Geometry: see drawing. Coordinates: mm, zero at the bounding-box minimum. A direction names the side the tool comes from. Round coordinates to 2 decimals unless told otherwise and drop trailing zeros. Loops run counter-clockwise (first coordinate to the right, second up) from the corner with the lowest first, then second, coordinate; pieces in that order, holes last.
(1) Cut plane B-B, the plane y = 93.5. Output: boundary loops of the cut face in (x, z), and give its area (3 significant figures).
(2) Line query: line 1 (X direction, y = 96.5, z = 148); line 2 (X direction, y = 173, z = 15); line 3 (Y direction, x = 136, z = 57.5). Output: solid intervals per line, ascending.
(3) Access query for the marked faces 1, 2, 3 and 4. Directions: +Z, -Z, +X, -X, +Y, -Y. A direction counts if a zero-diameter tool reaches every point of the face in a straight line with its end or side. Return the directions, or none.
(4) Cut plane C-C, the plane x = 85. Output: boundary loops of the cut face in (y, z), and give its area (3 significant figures).
(5) First-contact query: pin 1 Ø10 at (y, z) = (62.5, 78) entering from +X; pin 2 Ø6 at (x, z) = (204.5, 25) entering from -Y; pin 3 Ø4 at (x, z) = (191.5, 154) entering from -Y. Flat tips, straight axial feed; report the tip coordinate or a pass-through.
(6) Cut plane A-A, the plane z = 51. Output: boundary loops of the cut face in (x, y), and give its area (3 significant figures).
(7) Cut plane D-D, the plane z = 92.5. Output: boundary loops of the cut face in (x, y), and give its area (3 significant figures).
(8) Draft query along X for the marked faces 5, 6, 7 and 8. Return one class per face: released by +X, released by -X, zero draft, split by the parting line, or undercut.
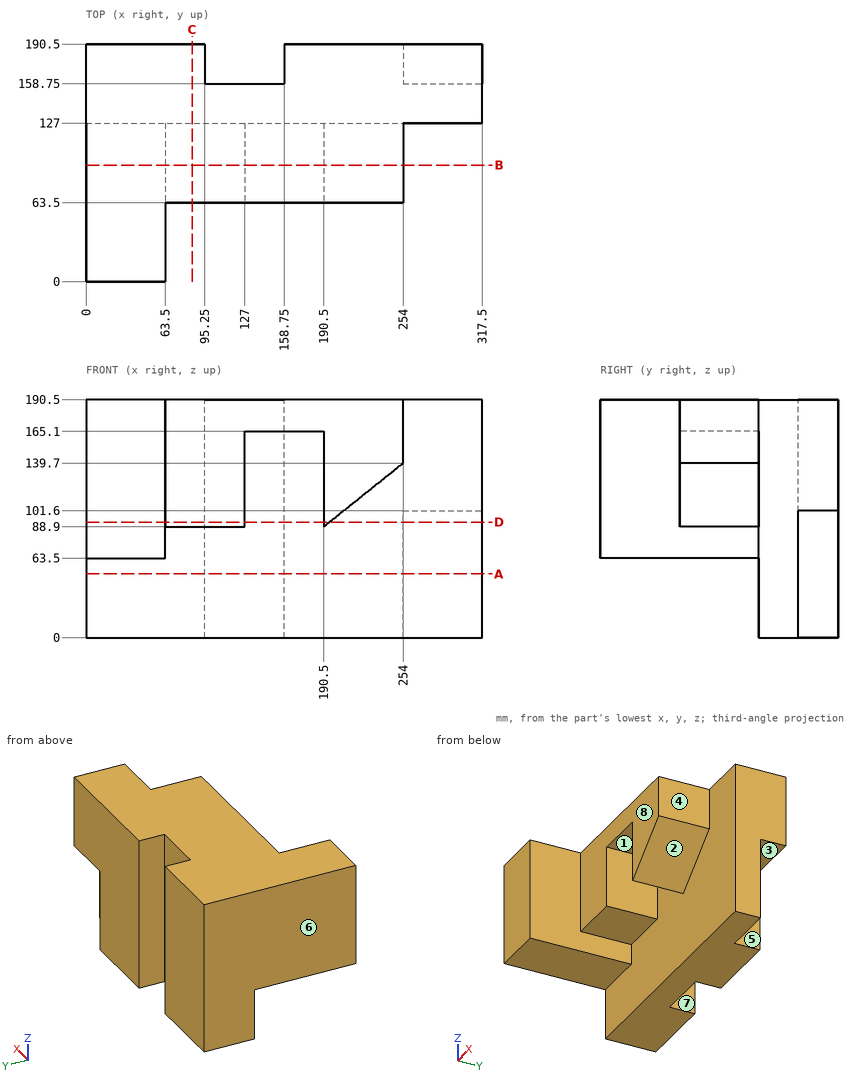
Reported:
1. outline: (0, 63.5) - (63.5, 63.5) - (63.5, 88.9) - (127, 88.9) - (127, 165.1) - (190.5, 165.1) - (190.5, 88.9) - (254, 139.7) - (254, 190.5) - (0, 190.5) - close
1. area: 21,000 mm2
2. line 1: x = 0 to 127, 190.5 to 254
2. line 2: x = 0 to 95.25, 158.75 to 254
2. line 3: y = 127 to 158.75
3. face 1: -Z, -Y
3. face 2: -Z, +X, -Y
3. face 3: -Z, +X, +Y
3. face 4: +Z, -Z, +X, -Y
4. outline: (63.5, 88.9) - (127, 88.9) - (127, 0) - (190.5, 0) - (190.5, 190.5) - (63.5, 190.5) - close
4. area: 18,500 mm2
5. pin 1: stops at x = 63.5
5. pin 2: stops at y = 127
5. pin 3: stops at y = 63.5
6. outline: (0, 127) - (317.5, 127) - (317.5, 158.75) - (254, 158.75) - (254, 190.5) - (158.75, 190.5) - (158.75, 158.75) - (95.25, 158.75) - (95.25, 190.5) - (0, 190.5) - close
6. area: 16,100 mm2
7. outline: (0, 0) - (63.5, 0) - (63.5, 63.5) - (127, 63.5) - (127, 127) - (190.5, 127) - (190.5, 63.5) - (195, 63.5) - (195, 127) - (317.5, 127) - (317.5, 158.75) - (254, 158.75) - (254, 190.5) - (158.75, 190.5) - (158.75, 158.75) - (95.25, 158.75) - (95.25, 190.5) - (0, 190.5) - close
7. area: 28,500 mm2
8. face 5: released by +X
8. face 6: released by -X
8. face 7: undercut
8. face 8: zero draft
